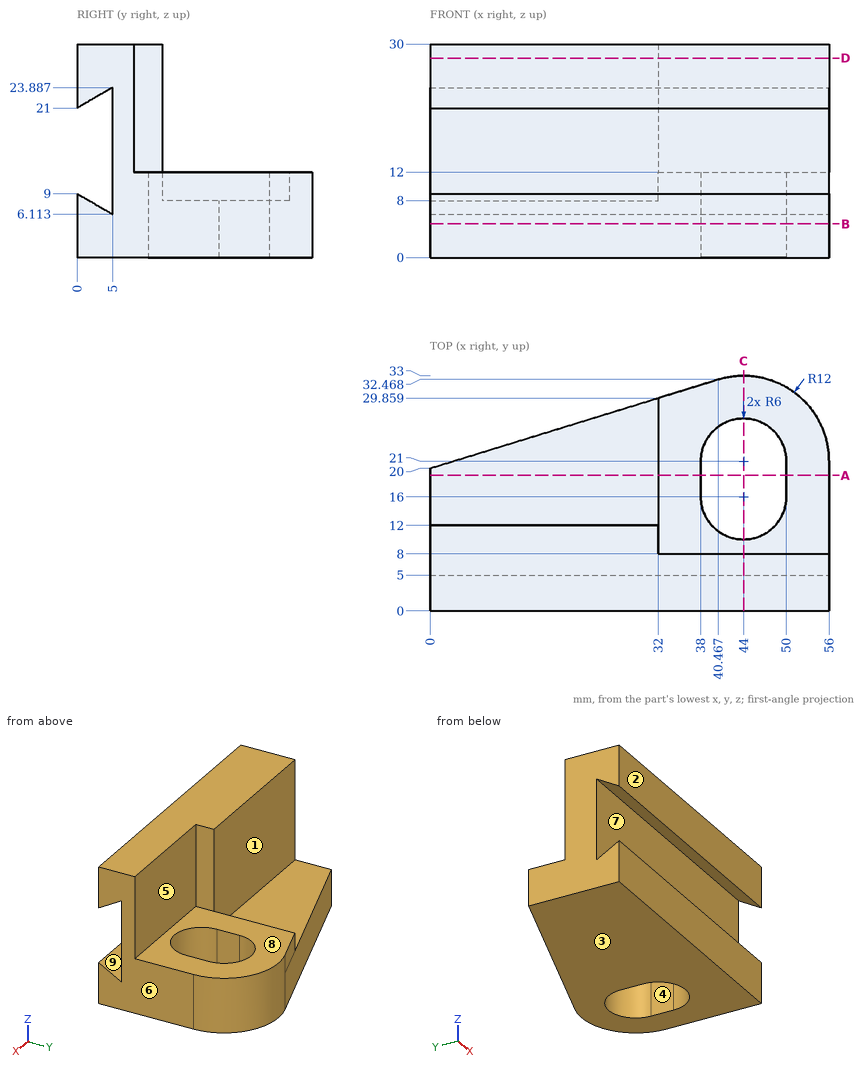
Input: dimensioned drawing with shaded views. Units: mm. Origin: part minimum x, y, z. A direction names the side the tool comes from. Round coordinates to 2 decimals unless told otherwise and drop trailing zeros. Loops run counter-clockwise (first coordinate to the right, second up) from the corner with the lowest first, then second, coordinate; pieces in that order, holes last.
1) Section query B-B on z = 4.75. Return the cut outline in (x, y).
Ans:
outline: (0, 0) - (56, 0) - (56, 21) arc R12 ccw to (40.47, 32.47) - (0, 20) - close; hole (38, 16) arc R6 ccw to (50, 16) - (50, 21) arc R6 ccw to (38, 21) - close
2) Pull-direction query (Z, two-part tool) for the marked faces 6, 7, 8 and 9; classes: released by +Z, released by -Z, zero draft, split by the parting line, or undercut.
Ans:
face 6: zero draft
face 7: undercut
face 8: released by +Z
face 9: undercut
3) Section query D-D on z = 28. Return the cut outline in (x, y), plus the area to 3 significant figures.
Ans:
outline: (0, 0) - (56, 0) - (56, 8) - (32, 8) - (32, 12) - (0, 12) - close
area: 576 mm2
4) Pin query (flat end, axial travel): pin 1 (8 mm diameter, centred on x = 25.5, z = 25, fed in from +Y); pin 2 (3 mm diameter, centred on y = 11, z = 21.5, fed in from +X); pin 3 (9 mm diameter, centred on x = 45.5, z = 20.5, fed in from +Y); pin 4 (6 mm diameter, centred on x = 45.5, y = 21, fed in from +Z). Return the tip coordinate at first contact, or that it passes through.
Ans:
pin 1: stops at y = 12
pin 2: stops at x = 32
pin 3: stops at y = 8
pin 4: passes through
5) Section query A-A on y = 19. Return the cut outline in (x, z).
Ans:
outline: (0, 0) - (38, 0) - (38, 12) - (32, 12) - (32, 8) - (0, 8) - close; (50, 0) - (56, 0) - (56, 12) - (50, 12) - close
6) Material intervals for line 1 (X direction, y = 18, z = 3.75); line 2 (Z direction, x = 49, y = 28.5); line 3 (Y direction, x = 39.5, z = 27.25), sorted ascending.
Ans:
line 1: x = 0 to 38, 50 to 56
line 2: z = 0 to 12
line 3: y = 0 to 8
7) Set-up query: the marked faces 1, 2, 3, 4 and 5. Return all of +Z, -Z, +X, -X, +Y, -Y with unobstructed straight access to the full face (end or side cutting, diameter ignored); none if empty.
Ans:
face 1: +Z, -X, +Y
face 2: +Z, -Z, +X, -X, -Y
face 3: -Z, +X, -X, +Y, -Y
face 4: +Z, -Z
face 5: +Z, +X, +Y
8) Section query C-C on x = 44. Return the cut outline in (y, z).
Ans:
outline: (0, 0) - (10, 0) - (10, 12) - (8, 12) - (8, 30) - (0, 30) - (0, 21) - (5, 23.89) - (5, 6.11) - (0, 9) - close; (27, 0) - (33, 0) - (33, 12) - (27, 12) - close
